The listing builds one solid part. Answer for the finished solid, in the listing's coordinates (mm). Give positions to 0.01 mm unless a question says otherwise; leave off trailing zeros. Loops run counter-clockwise (first coordinate to the right, second up) from the corner with the lowest first, then second, coordinate; pieces in that order, holes last.
Item 1: Section C-C, the plane z = 37 is taken. Give the vertices of the cut face in (x, y), and give its area (3 significant figures).
Item 2: The mould has two halves that part along Z. Classify faces 1 (the face through (32, -1, 23)), 2 (the face through (-7.723, -0.986, 27.973)), 3 (the face through (31, -1, 73)): pulls with the +Z half, pulls with the -Z half, needs draft (parallel to the pull), parting line crosses it, or undercut.
Item 3: Each of these flat-tipped pins is pushed along its axis until it touches: pin 1 Ø3 at (x, z) = (8, 37) entering from -Y; pin 2 Ø1.6 at (x, z) = (0, 45) entering from +Y. Where does it stop, or does it pass through?
Item 4: Section D-D, the plane x = 0 is taken. Give the vertices of the cut face in (y, z).
Item 5: Section A-A, the plane z = 67 is taken. Give the vertices of the cut face in (x, y).
Item 6: Consider line 1 along X through (y, z) = (-1.1, 37); line 2 along X through (y, z) = (-0.65, 67); line 3 along X through (y, z) = (-1.1, 29). Determine where each line is inside the solid, lowest interval first.
Item 7: Section B-B, the plane x = -25 is taken. Give the vertices of the cut face in (y, z), and give its area (3 significant figures).
from build123d import *

# Parameters (mm, degrees)
SKETCH1_W          = 64
SKETCH1_H          = 2
BASE_FLANGE1_DEPTH = 74
SKETCH2_R          = 1.75
CUT_EXTRUDE1_DEPTH = 10
CUT_EXTRUDE2_REACH = 82.647
SKETCH4_R          = 4
CHAMFER1_SIZE      = 2
CUT_EXTRUDE5_REACH = 82.647
SKETCH7_R          = 1
SKETCH7_R_2        = 1.25
SKETCH8_W          = 64
SKETCH8_H          = 30
TAB1_DEPTH         = 2
CHAMFER2_SIZE      = 2


# Sheet-metal steps are written as plain solids
with BuildPart() as part:
    # Sketch1 → Base-Flange1 (new body)
    with BuildSketch(Plane.XY):
        with Locations((0, -1)):
            Rectangle(SKETCH1_W, SKETCH1_H)
    extrude(amount=BASE_FLANGE1_DEPTH)

    # Sketch2 → Cut-Extrude1 (cut)
    with BuildSketch(Plane(origin=(0, 0, 0), x_dir=(1, 0, 0), z_dir=(0, 1, 0))):
        with Locations(Location((-25, -7, 0), (0, 0, 270))):
            Circle(SKETCH2_R)
        with Locations(Location((-25, -67, 0), (0, 0, 270))):
            Circle(SKETCH2_R)
        with Locations(Location((25, -67, 0), (0, 0, 270))):
            Circle(SKETCH2_R)
        with Locations(Location((25, -7, 0), (0, 0, 270))):
            Circle(SKETCH2_R)
    extrude(amount=-CUT_EXTRUDE1_DEPTH, mode=Mode.SUBTRACT)

    # Sketch4 → Cut-Extrude2 (cut, up to next)
    with BuildSketch(Plane(origin=(0, 0, 0), x_dir=(1, 0, 0), z_dir=(0, 1, 0)), mode=Mode.PRIVATE) as cut_extrude2_sk1:
        with Locations(Location((0, -37, 0), (0, 0, 270))):
            Circle(SKETCH4_R)
    cut_extrude2_tool1 = extrude(cut_extrude2_sk1.sketch, amount=-CUT_EXTRUDE2_REACH, mode=Mode.PRIVATE) & part.part
    add(cut_extrude2_tool1.solids().sort_by_distance((0, 0, 37))[0], mode=Mode.SUBTRACT)

    # Chamfer1
    chamfer1_edges = [part.edges().sort_by_distance(p)[0] for p in [
        (-32, -1, 74),
        (32, -1, 74),
    ]]
    chamfer(chamfer1_edges, length=CHAMFER1_SIZE)

    # Sketch7 → Cut-Extrude5 (cut, up to next)
    with BuildSketch(Plane(origin=(0, 0, 0), x_dir=(1, 0, 0), z_dir=(0, 1, 0)), mode=Mode.PRIVATE) as cut_extrude5_sk1:
        with Locations(Location((-8, -37, 0), (0, 0, 270))):
            Circle(SKETCH7_R)
    cut_extrude5_tool1 = extrude(cut_extrude5_sk1.sketch, amount=-CUT_EXTRUDE5_REACH, mode=Mode.PRIVATE) & part.part
    # Sketch7 → Cut-Extrude5 (cut, up to next)
    with BuildSketch(Plane(origin=(0, 0, 0), x_dir=(1, 0, 0), z_dir=(0, 1, 0)), mode=Mode.PRIVATE) as cut_extrude5_sk2:
        with Locations(Location((8, -37, 0), (0, 0, 270))):
            Circle(SKETCH7_R)
    cut_extrude5_tool2 = extrude(cut_extrude5_sk2.sketch, amount=-CUT_EXTRUDE5_REACH, mode=Mode.PRIVATE) & part.part
    # Sketch7 → Cut-Extrude5 (cut, up to next)
    with BuildSketch(Plane(origin=(0, 0, 0), x_dir=(1, 0, 0), z_dir=(0, 1, 0)), mode=Mode.PRIVATE) as cut_extrude5_sk3:
        with Locations(Location((0, -45, 0), (0, 0, 270))):
            Circle(SKETCH7_R)
    cut_extrude5_tool3 = extrude(cut_extrude5_sk3.sketch, amount=-CUT_EXTRUDE5_REACH, mode=Mode.PRIVATE) & part.part
    # Sketch7 → Cut-Extrude5 (cut, up to next)
    with BuildSketch(Plane(origin=(0, 0, 0), x_dir=(1, 0, 0), z_dir=(0, 1, 0)), mode=Mode.PRIVATE) as cut_extrude5_sk4:
        with Locations(Location((0, -29, 0), (0, 0, 270))):
            Circle(SKETCH7_R)
    cut_extrude5_tool4 = extrude(cut_extrude5_sk4.sketch, amount=-CUT_EXTRUDE5_REACH, mode=Mode.PRIVATE) & part.part
    # Sketch7 → Cut-Extrude5 (cut, up to next)
    with BuildSketch(Plane(origin=(0, 0, 0), x_dir=(1, 0, 0), z_dir=(0, 1, 0)), mode=Mode.PRIVATE) as cut_extrude5_sk5:
        with Locations(Location((-7.778174593, -44.778174593, 0), (0, 0, 270))):
            Circle(SKETCH7_R_2)
    cut_extrude5_tool5 = extrude(cut_extrude5_sk5.sketch, amount=-CUT_EXTRUDE5_REACH, mode=Mode.PRIVATE) & part.part
    # Sketch7 → Cut-Extrude5 (cut, up to next)
    with BuildSketch(Plane(origin=(0, 0, 0), x_dir=(1, 0, 0), z_dir=(0, 1, 0)), mode=Mode.PRIVATE) as cut_extrude5_sk6:
        with Locations(Location((-7.778174593, -29.221825407, 0), (0, 0, 270))):
            Circle(SKETCH7_R_2)
    cut_extrude5_tool6 = extrude(cut_extrude5_sk6.sketch, amount=-CUT_EXTRUDE5_REACH, mode=Mode.PRIVATE) & part.part
    # Sketch7 → Cut-Extrude5 (cut, up to next)
    with BuildSketch(Plane(origin=(0, 0, 0), x_dir=(1, 0, 0), z_dir=(0, 1, 0)), mode=Mode.PRIVATE) as cut_extrude5_sk7:
        with Locations(Location((7.778174593, -29.221825407, 0), (0, 0, 270))):
            Circle(SKETCH7_R_2)
    cut_extrude5_tool7 = extrude(cut_extrude5_sk7.sketch, amount=-CUT_EXTRUDE5_REACH, mode=Mode.PRIVATE) & part.part
    # Sketch7 → Cut-Extrude5 (cut, up to next)
    with BuildSketch(Plane(origin=(0, 0, 0), x_dir=(1, 0, 0), z_dir=(0, 1, 0)), mode=Mode.PRIVATE) as cut_extrude5_sk8:
        with Locations(Location((7.778174593, -44.778174593, 0), (0, 0, 270))):
            Circle(SKETCH7_R_2)
    cut_extrude5_tool8 = extrude(cut_extrude5_sk8.sketch, amount=-CUT_EXTRUDE5_REACH, mode=Mode.PRIVATE) & part.part
    add(cut_extrude5_tool1.solids().sort_by_distance((-8, 0, 37))[0], mode=Mode.SUBTRACT)
    add(cut_extrude5_tool2.solids().sort_by_distance((8, 0, 37))[0], mode=Mode.SUBTRACT)
    add(cut_extrude5_tool3.solids().sort_by_distance((0, 0, 45))[0], mode=Mode.SUBTRACT)
    add(cut_extrude5_tool4.solids().sort_by_distance((0, 0, 29))[0], mode=Mode.SUBTRACT)
    add(cut_extrude5_tool5.solids().sort_by_distance((-7.778175, 0, 44.778175))[0], mode=Mode.SUBTRACT)
    add(cut_extrude5_tool6.solids().sort_by_distance((-7.778175, 0, 29.221825))[0], mode=Mode.SUBTRACT)
    add(cut_extrude5_tool7.solids().sort_by_distance((7.778175, 0, 29.221825))[0], mode=Mode.SUBTRACT)
    add(cut_extrude5_tool8.solids().sort_by_distance((7.778175, 0, 44.778175))[0], mode=Mode.SUBTRACT)

    # Sketch8 → Tab1 (add)
    with BuildSketch(Plane(origin=(0, 0, 0), x_dir=(1, 0, 0), z_dir=(0, 1, 0))):
        with Locations((0, 15)):
            Rectangle(SKETCH8_W, SKETCH8_H)
    extrude(amount=-TAB1_DEPTH)

    # Chamfer2
    chamfer2_edges = [part.edges().sort_by_distance(p)[0] for p in [
        (-32, -1, -30),
        (32, -1, -30),
    ]]
    chamfer(chamfer2_edges, length=CHAMFER2_SIZE)


solid = part.part
Worked answers:
1. outline: (-32, -2) - (-9, -2) - (-9, 0) - (-32, 0) - close; (-7, -2) - (-4, -2) - (-4, 0) - (-7, 0) - close; (4, -2) - (7, -2) - (7, 0) - (4, 0) - close; (9, -2) - (32, -2) - (32, 0) - (9, 0) - close
1. area: 104 mm2
2. face 1: needs draft
2. face 2: undercut
2. face 3: pulls with the +Z half
3. pin 1: stops at y = -2
3. pin 2: passes through
4. outline: (-2, -30) - (0, -30) - (0, 28) - (-2, 28) - close; (-2, 30) - (0, 30) - (0, 33) - (-2, 33) - close; (-2, 41) - (0, 41) - (0, 44) - (-2, 44) - close; (-2, 46) - (0, 46) - (0, 74) - (-2, 74) - close
5. outline: (-32, -2) - (-26.75, -2) - (-26.75, 0) - (-32, 0) - close; (-23.25, -2) - (23.25, -2) - (23.25, 0) - (-23.25, 0) - close; (26.75, -2) - (32, -2) - (32, 0) - (26.75, 0) - close
6. line 1: x = -32 to -9, -7 to -4, 4 to 7, 9 to 32
6. line 2: x = -32 to -26.75, -23.25 to 23.25, 26.75 to 32
6. line 3: x = -32 to -9.01, -6.55 to -1, 1 to 6.55, 9.01 to 32
7. outline: (-2, -30) - (0, -30) - (0, 5.25) - (-2, 5.25) - close; (-2, 8.75) - (0, 8.75) - (0, 65.25) - (-2, 65.25) - close; (-2, 68.75) - (0, 68.75) - (0, 74) - (-2, 74) - close
7. area: 194 mm2
